Verification items for the finished model (mm, model axes). A direction names the side the tool comes from. Coordinates: 2 decimals unless noted, no trailing zeros. Order: outer loops, then holes, each group sorted by start corner. A loop starts at its lowest first (then second) coordinate and runs counter-clockwise, first axis right, second up. Notation, with made-up numbers: (-35, 68) -> (-12, 68) arc R6 cw to (-12, 74) -> close; hole circle Ø6 at (31, -7.5). An arc over 180 degrees is marked (long way). Write item = value, one per line. Start each with the question number.
1. Cross-section at A-A on y = 7.5. Record the cut outline in (x, z), plus the area to 3 significant figures.
2. Go/stop test with flat-tipped pins: P1, Ø3.5, axis at x = 5, y = 7.5, coming from the +Z side; P2, Ø5, axis at x = 17.5, y = 10, coming from the +Z side; P3, Ø1, axis at y = 4.5, z = 5.5, coming from the +X side; P4, Ø7, axis at x = 30, y = 7.5, coming from the +Z side. Record where each tip stops, or that it passes through.
3. Set-up check for faces 1 (the flat face through (17, 0, 2)), 2 (the flat face through (17, 8, 7)): record each of +Z, -Z, +X, -X, +Y, -Y from which the full face is reachable in a straight line by a thin tool's end or side.
4. Cross-section at D-D on x = 11.5. Record the cut outline in (y, z).
5. Release check for a two-part mould opening along Y. For faces 3 (the cylindrical face through (6.183, 9.355, 1.972)), 4 (the cylindrical face through (2, 14, 2)), 5 (the flat face through (8, 8, 0)) record: +Y half, -Y half, draft (parallel to the pull), parting line (faces both ways), or undercut.
6. Cross-section at C-C on x = 29.5. Record the cut outline in (y, z), plus the area to 3 significant figures.
7. Cross-section at B-B on z = 2. Record the cut outline in (x, y).
8. Thickness scan on line 1 along Y through (x, z) = (5, 2.7); line 2 along X through (y, z) = (7, 0.5); line 3 along Z through (x, y) = (20, 3.75). Record the ranges inside material, lowest first. Write a range as from..to.
from build123d import *

# Parameters (mm, degrees)
CROQUIS1_W              = 35
CROQUIS1_H              = 15
CROQUIS1_R              = 2.2
SALIENTE_EXTRUIR1_DEPTH = 4
CROQUIS2_R              = 7.5
CROQUIS2_R_2            = 5.25
SALIENTE_EXTRUIR2_DEPTH = 5
REDONDEO1_R             = 5
CROQUIS3_R              = 0.6
CORTAR_EXTRUIR1_DEPTH   = 32
CROQUIS4_R              = 5.25
SALIENTE_EXTRUIR3_DEPTH = 3


with BuildPart() as part:
    # Croquis1 → Saliente-Extruir1 (new body)
    with BuildSketch(Plane.XY):
        with Locations((17.5, 7.5)):
            Rectangle(CROQUIS1_W, CROQUIS1_H)
        with Locations((5, 7.5)):
            Circle(CROQUIS1_R, mode=Mode.SUBTRACT)
        with Locations((30, 7.5)):
            Circle(CROQUIS1_R, mode=Mode.SUBTRACT)
    extrude(amount=SALIENTE_EXTRUIR1_DEPTH)

    # Croquis2 → Saliente-Extruir2 (add)
    with BuildSketch(Plane.XY.offset(4)):
        with Locations(Location((17.5, 7.5, 0), (0, 0, 270))):
            Circle(CROQUIS2_R)
        with Locations((17.5, 7.5)):
            Circle(CROQUIS2_R_2, mode=Mode.SUBTRACT)
    extrude(amount=SALIENTE_EXTRUIR2_DEPTH)

    # Redondeo1
    redondeo1_edges = [part.edges().sort_by_distance(p)[0] for p in [
        (0, 0, 2),
        (0, 15, 2),
        (35, 15, 2),
        (35, 0, 2),
    ]]
    fillet(redondeo1_edges, radius=REDONDEO1_R)

    # Croquis3 → Cortar-Extruir1 (cut)
    with BuildSketch(Plane(origin=(0, 15, 0), x_dir=(1, 0, 0), z_dir=(0, 1, 0))):
        with Locations((17.5, 0)):
            Circle(CROQUIS3_R)
    extrude(amount=-CORTAR_EXTRUIR1_DEPTH, mode=Mode.SUBTRACT)

    # Croquis4 → Saliente-Extruir3 (add)
    with BuildSketch(Plane.XY.offset(4)):
        with Locations((17.5, 7.5)):
            Circle(CROQUIS4_R)
    extrude(amount=SALIENTE_EXTRUIR3_DEPTH)


solid = part.part
Worked out:
q1.outline = (0, 0) -> (2.8, 0) -> (2.8, 4) -> (0, 4) -> close; (7.2, 0) -> (16.9, 0) arc R0.6 cw to (18.1, 0) -> (27.8, 0) -> (27.8, 4) -> (25, 4) -> (25, 9) -> (22.75, 9) -> (22.75, 7) -> (12.25, 7) -> (12.25, 9) -> (10, 9) -> (10, 4) -> (7.2, 4) -> close; (32.2, 0) -> (35, 0) -> (35, 4) -> (32.2, 4) -> close
q1.area = 158 mm²
q2.P1 = through
q2.P2 = 7
q2.P3 = 24.57
q2.P4 = 4
q3.face_1 = +Z, -Z, +X, -X, -Y
q3.face_2 = +Z
q4.outline = (0, 0) -> (15, 0) -> (15, 4) -> (12, 4) -> (12, 9) -> (3, 9) -> (3, 4) -> (0, 4) -> close
q5.face_3 = undercut
q5.face_4 = +Y half
q5.face_5 = draft
q6.outline = (0, 0) -> (5.36, 0) -> (5.36, 4) -> (0, 4) -> close; (9.64, 0) -> (15, 0) -> (15, 4) -> (9.64, 4) -> close
q6.area = 42.9 mm²
q7.outline = (0, 5) arc R5 ccw to (5, 0) -> (30, 0) arc R5 ccw to (35, 5) -> (35, 10) arc R5 ccw to (30, 15) -> (5, 15) arc R5 ccw to (0, 10) -> close; hole circle Ø4.4 at (5, 7.5); hole circle Ø4.4 at (30, 7.5)
q8.line_1 = 0..5.3, 9.7..15
q8.line_2 = 0..2.86, 7.14..17.17, 17.83..27.86, 32.14..35
q8.line_3 = 0..7
